```python
from build123d import *

# Parameters (mm, degrees)
EXTRUDE_1_DEPTH     = 12
CUT_EXTRUDE_1_REACH = 111.567
SKETCH_3_R          = 3


with BuildPart() as part:
    # 草图2 → 凸台-拉伸1 (new body)
    with BuildSketch(Plane(origin=(0, 0, 0), x_dir=(0, 0, -1), z_dir=(1, 0, 0))):
        Polygon((-53, 0), (53, 0), (53, 20), (53, 22), (89, 22), (89, 25), (50, 25), (50, 20), (50, 3), (-50, 3), (-50, 14), (-53, 14), align=None)
    extrude(amount=EXTRUDE_1_DEPTH)

    # 切除-拉伸1: up to this face of the body (flat: up to its plane)
    cut_extrude_1_end = Plane(part.part.faces().sort_by_distance((6, 7, 53))[0])
    # 草图3 → 切除-拉伸1 (cut, up to the picked face)
    with BuildSketch(Plane(origin=(0, 0, -53), x_dir=(-1, 0, 0), z_dir=(0, 0, -1)), mode=Mode.PRIVATE) as cut_extrude_1_sk1:
        with Locations((-6, 14)):
            Circle(SKETCH_3_R)
    cut_extrude_1_tool1 = split(extrude(cut_extrude_1_sk1.sketch, amount=-CUT_EXTRUDE_1_REACH, mode=Mode.PRIVATE), bisect_by=cut_extrude_1_end, keep=Keep.BOTH, mode=Mode.PRIVATE)
    add(cut_extrude_1_tool1.solids().sort_by(Axis((6, 14, -53), (0, 0, 1)))[0], mode=Mode.SUBTRACT)


solid = part.part
```
Geometry: final body of the model. Coordinates: model frame, mm. A direction names the side the tool comes from. Round coordinates to 2 decimals unless told otherwise and drop trailing zeros. Order: outer loops, then holes, each group sorted by start corner. A loop starts at its lowest first (then second) coordinate and runs counter-clockwise, first axis right, second up. Notation, with made-up numbers: M -17,-4.75 L -9,-4.75 A28 cw -9,15.25 Z; hole C 13,20 d9. An arc over 180 degrees is marked long. Use one line per item in the form item = value. Start each with the question number.
Q1. Mould query, pull axis X, two halves, no side actions, for faces 1 (the face through (6, 11, 51)), 2 (the face through (10, 14, 51)), 3 (the face through (12, 2, -7)). Classes: +X half, -X half, draft (parallel to the pull), parting line (faces both ways), or undercut.
Q2. Access query for faces 4 (the face through (6, 3, -1)), 5 (the face through (4.616, 11.338, -51.521)), 6 (the face through (6, 23, -89)), 7 (the face through (1, 14, 51)), 8 (the face through (6, 22, -71)). Directions: +Z, -Z, +X, -X, +Y, -Y. A direction counts if a zero-diameter tool reaches every point of the face in a straight line with its end or side. Return the directions, or none.
Q3. Pin query (flat end, axial travel): pin 1 Ø3.5 at (x, y) = (6, 14) entering from -Z; pin 2 Ø3.5 at (x, z) = (2, 51) entering from +Y; pin 3 Ø3.5 at (x, y) = (9, 6) entering from -Z; pin 4 Ø1.5 at (x, z) = (7.5, -20) entering from +Y. Return the tip coordinate at first contact, or that it passes through.
Q4. Cut plane B-B (y = 5.5). Return loops of the section in (x, z).
Q5. Cut plane A-A (x = 6). Return loops of the section in (y, z).
Q6. Material intervals for line 1 (Y direction, x = 6, z = -51.7); line 2 (Z direction, x = 6, y = 9.75); line 3 (Y direction, x = 4.5, z = -55.5), sorted ascending. Write a range as [from, to].
Q7. Cut plane C-C (z = -19). Return loops of the section in (x, y).
Geometry results:
q1.face_1 = undercut
q1.face_2 = draft
q1.face_3 = +X half
q2.face_4 = +X, -X, +Y
q2.face_5 = +Z, -Z
q2.face_6 = -Z, +X, -X, +Y, -Y
q2.face_7 = +Z, +X, -X, +Y
q2.face_8 = -Z, +X, -X, -Y
q3.pin_1 = through
q3.pin_2 = 14
q3.pin_3 = -53
q3.pin_4 = 3
q4.outline = M 0,-53 L 12,-53 L 12,-50 L 0,-50 Z; M 0,50 L 12,50 L 12,53 L 0,53 Z
q5.outline = M 0,-53 L 11,-53 L 11,-50 L 3,-50 L 3,50 L 11,50 L 11,53 L 0,53 Z; M 17,-53 L 22,-53 L 22,-89 L 25,-89 L 25,-50 L 17,-50 Z
q6.line_1 = [0, 11], [17, 25]
q6.line_2 = [-53, -50], [50, 53]
q6.line_3 = [22, 25]
q7.outline = M 0,0 L 12,0 L 12,3 L 0,3 Z
